Design review of the part shown in the three views and the two pictorial views. Dimensions are in mm from the part's minimum x, y and z. Round coordinates to 2 decimals unless told otherwise and drop trailing zeros. Write each loop counter-clockwise with the first axis right and the second up, starting at its lowest first coordinate (ties: lowest second). Pieces come first, ordered by that corner, then holes. Notation, with made-up numbers: (60, 16) -> (117, 16) arc R16 ccw to (117, 41) -> close; hole circle Ø3 at (4, -11.75). An arc over 180 degrees is marked (long way). One line per question, with ' | ' between items. Start each with the question number.
1) Consider section D-D (z = 1.15). Give the boundary of the cut face in (x, y).
2) For probe 1 along Y at (x, z) = (69.5, 0.95); probe 2 along X at (y, z) = (89, 2.4); probe 3 along Y at (x, z) = (3.5, 0.55), list the stretches that pass through material, from the lowest coordinate up.
3) Consider section C-C (y = 86). Give the boundary of the cut face in (x, z).
4) Consider section B-B (x = 5.5). Give the boundary of the cut face in (y, z), then the cut area to 3 significant figures.
5) Consider section A-A (y = 14.75). Give the boundary of the cut face in (x, z).
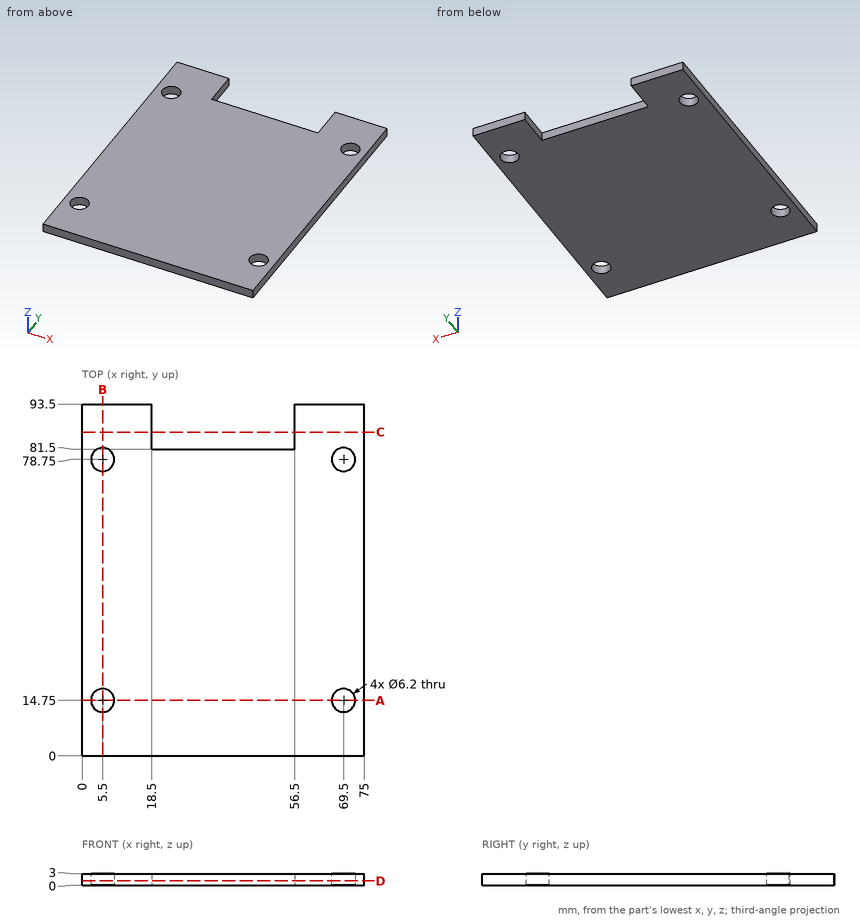
From the geometry:
1) outline: (0, 0) -> (75, 0) -> (75, 93.5) -> (56.5, 93.5) -> (56.5, 81.5) -> (18.5, 81.5) -> (18.5, 93.5) -> (0, 93.5) -> close; hole circle Ø6.2 at (5.5, 14.75); hole circle Ø6.2 at (5.5, 78.75); hole circle Ø6.2 at (69.5, 14.75); hole circle Ø6.2 at (69.5, 78.75)
2) probe 1: y = 0 to 11.65, 17.85 to 75.65, 81.85 to 93.5 | probe 2: x = 0 to 18.5, 56.5 to 75 | probe 3: y = 0 to 12.38, 17.12 to 76.38, 81.12 to 93.5
3) outline: (0, 0) -> (18.5, 0) -> (18.5, 3) -> (0, 3) -> close; (56.5, 0) -> (75, 0) -> (75, 3) -> (56.5, 3) -> close
4) outline: (0, 0) -> (11.65, 0) -> (11.65, 3) -> (0, 3) -> close; (17.85, 0) -> (75.65, 0) -> (75.65, 3) -> (17.85, 3) -> close; (81.85, 0) -> (93.5, 0) -> (93.5, 3) -> (81.85, 3) -> close | area: 243 mm2
5) outline: (0, 0) -> (2.4, 0) -> (2.4, 3) -> (0, 3) -> close; (8.6, 0) -> (66.4, 0) -> (66.4, 3) -> (8.6, 3) -> close; (72.6, 0) -> (75, 0) -> (75, 3) -> (72.6, 3) -> close
